CAD build for the part. Positions are in the model's coordinates, mm. A direction names the side the tool comes from. Round coordinates to 2 decimals unless told otherwise and drop trailing zeros. Write each loop counter-clockwise with the first axis right and the second up, starting at its lowest first coordinate (ties: lowest second). Pieces come first, ordered by that corner, then holes. Notation, with made-up numbers: (71.25, 1.25) - (86.25, 1.25) arc R13 ccw to (86.25, 9.25) - close; hole circle Ø9 at (-7.5, 19). An arc over 180 degrees is marked (long way). Put each result on its own line as item: value. Start each with the question number.
Item 1: Cut at A-A (x = -14.5). Give the cut face in (y, z).
Item 2: Drill centre lines: line 1 (Y direction, x = 0, z = 31.5); line 2 (Z direction, x = 3, y = 5.5); line 3 (Z direction, x = -17, y = 9.5). Where is each one in solid material? Low to high. Write a range as from..to.
Item 3: Cut at B-B (y = 10.5). Give the cut face in (x, z), and give its area (3 significant figures).
Item 4: Pin check, flat tips, straight feed: pin 1 Ø3 at (y, z) = (5, 20) entering from +X; pin 2 Ø8 at (y, z) = (14.5, 6.5) entering from -X; pin 3 Ø10 at (x, y) = (-5.5, 12.5) entering from +Z. Stop position of each tip, or through.
Item 5: Cut at C-C (z = 7). Give the cut face in (x, y).
Item 6: 3-axis set-ups, long thin cutter, end or side, ignore diameter. For faces 1 (the flat face through (0, 10, 5)), 2 (the flat face through (8, 8, 30)), 3 (the cylindrical face through (9.229, -17.743, 19.72)), 4 (the flat face through (0, 10, 25)), 5 (the flat face through (4, -4, 0)): which of +Z, -Z, +X, -X, +Y, -Y reach the whole face in a straight line?
Item 7: Cut at D-D (x = 9.5). Give the cut face in (y, z).
```python
from build123d import *

# Parameters (mm, degrees)
SKETCH2_R               = 20
BOSS_EXTRUDE1_DEPTH     = 40
SKETCH3_W               = 10
SKETCH3_H               = 20
CUT_EXTRUDE1_DEPTH      = 40
CUT_EXTRUDE1_DEPTH_BACK = 40
CUT_EXTRUDE2_DEPTH      = 10
CUT_EXTRUDE3_DEPTH      = 10


with BuildPart() as part:
    # Sketch2 → Boss-Extrude1 (new body)
    with BuildSketch(Plane.XY):
        Circle(SKETCH2_R)
    extrude(amount=BOSS_EXTRUDE1_DEPTH)

    # Sketch3 → Cut-Extrude1 (cut, two sides)
    with BuildSketch(Plane(origin=(0, 0, 0), x_dir=(0, 0, -1), z_dir=(1, 0, 0))) as cut_extrude1_sk:
        with Locations((-35, 10)):
            Rectangle(SKETCH3_W, SKETCH3_H)
    extrude(amount=CUT_EXTRUDE1_DEPTH, mode=Mode.SUBTRACT)
    extrude(cut_extrude1_sk.sketch, amount=-CUT_EXTRUDE1_DEPTH_BACK, mode=Mode.SUBTRACT)

    # Sketch4 → Cut-Extrude2 (cut)
    with BuildSketch(Plane.XY.offset(30)):
        with BuildLine():
            Line((0, 0), (0, 20))
            ThreePointArc((0, 20), (-14.142135624, 14.142135624), (-20, 0))
            Line((-20, 0), (0, 0))
        make_face()
    extrude(amount=-CUT_EXTRUDE2_DEPTH, mode=Mode.SUBTRACT)

    # Sketch5 → Cut-Extrude3 (cut)
    with BuildSketch(Plane(origin=(0, 0, 0), x_dir=(-1, 0, 0), z_dir=(0, 0, -1))):
        with BuildLine():
            Line((0, 20), (0, 0))
            Line((0, 0), (20, 0))
            ThreePointArc((20, 0), (14.142135624, 14.142135624), (0, 20))
        make_face()
    extrude(amount=-CUT_EXTRUDE3_DEPTH, mode=Mode.SUBTRACT)


solid = part.part
```
Output values:
1. outline: (-13.77, 0) - (0, 0) - (0, 10) - (13.77, 10) - (13.77, 20) - (0, 20) - (0, 40) - (-13.77, 40) - close
2. line 1: -20..0
2. line 2: 0..30
2. line 3: 10..20
3. outline: (-17.02, 10) - (0, 10) - (0, 0) - (17.02, 0) - (17.02, 30) - (0, 30) - (0, 20) - (-17.02, 20) - close
3. area: 681 mm2
4. pin 1: x = 19.69
4. pin 2: x = -15.56
4. pin 3: z = 20
5. outline: (-20, 0) arc R20 ccw (long way) to (0, 20) - (0, 0) - close
6. face 1: -Z, -X, +Y
6. face 2: +Z, +X, -X, +Y
6. face 3: +Z, -Z
6. face 4: +Z, -X, +Y
6. face 5: -Z, +X, -X, +Y, -Y
7. outline: (-17.6, 0) - (17.6, 0) - (17.6, 30) - (0, 30) - (0, 40) - (-17.6, 40) - close
